Here's how the part is built. I have some questions about the finished solid (model axes, mm). A direction names the side the tool comes from. Round coordinates to 2 decimals unless told otherwise and drop trailing zeros. Write each loop counter-clockwise with the first axis right and the second up, starting at its lowest first coordinate (ties: lowest second). Pieces come first, ordered by that corner, then holes. Notation, with made-up numbers: (65.25, 72) -> (82.25, 72) arc R23 cw to (82.25, 88) -> close; hole circle Ø4 at (-21.5, 38). An arc over 180 degrees is marked (long way). Put each result on its own line as item: value. Start each with the question number.
1) I want a section at A-A, the plane x = 28.5. List the corners of the cut face in (y, z) for me.
2) I want a section at C-C, the plane y = 7. List the corners of the cut face in (x, z) for me.
3) I want a section at D-D, the plane x = 16.5. List the corners of the cut face in (y, z) for me, then the cut area to 3 significant figures.
4) Which directions (+Z, -Z, +X, -X, +Y, -Y) give clear straight access to the entire face, cutting with the end or side of a thin tool? Please do faces 5 (the flat face through (24.088, -24, 2)), 6 (the flat face through (32.004, -19, 2)), 7 (the flat face through (30, 16.002, 2)), 8 (the flat face through (12.817, -23, 2)), 9 (the flat face through (19.202, 21, 2)).
5) Will these pins go through, and if not, where does the flat tip stop? P1, Ø1.4, axis at x = 26, z = 3, coming from the -Y side; P2, Ø1.6, axis at x = 6.5, z = 3, coming from the +Y side; P3, Ø1.4, axis at y = -12, z = 1.5, coming from the +X side.
6) We'd pull the mould along Y, two halves only. Please class faces 1 (the flat face through (5.98, -8, 2)), 2 (the flat face through (27.445, 11, 2)), 3 (the flat face through (30, 5.334, 2)), 4 (the flat face through (7, 3.272, 2)): released by +Y, released by -Y, zero draft, split by the parting line, or undercut.
7) If I drill on line 1 along Y through (x, z) = (29.25, 4.25); line 2 along X through (y, z) = (21, 1.45); line 3 along X through (y, z) = (-12, 0.3), over which ranges is the centre line in solid material (lowest first)? Write a range as [from, to].
8) I want a section at B-B, the plane z = 1.05. List the corners of the cut face in (x, y) for me.
from build123d import *

# Parameters (mm, degrees)
BOSS_EXTRUDE1_DEPTH = 4.5593


with BuildPart() as part:
    # Sketch1 → Boss-Extrude1 (new body)
    with BuildSketch(Plane.XY):
        Polygon((24.0884075, -21.336), (32.004, -21.336), (32.004, -16.002), (27.4447, -16.002), (27.4447, -5.334), (32.004, -5.334), (32.004, 5.334), (27.4447, 5.334), (27.4447, 16.002), (32.004, 16.002), (32.004, 26.67), (19.2024, 26.67), (19.2024, 21.336), (19.2024, 16.002), (7.47522, 16.002), (7.47522, 12.9921), (7.47522, 3.27152), (5.980176, 3.27152), (5.980176, -19.0119), (8.2572225, -19.0119), (12.8165225, -19.0119), (12.8165225, -26.67), (24.0884075, -26.67), align=None)
    extrude(amount=BOSS_EXTRUDE1_DEPTH)


solid = part.part
Findings:
1. outline: (-21.34, 0) -> (-16, 0) -> (-16, 4.56) -> (-21.34, 4.56) -> close; (-5.33, 0) -> (5.33, 0) -> (5.33, 4.56) -> (-5.33, 4.56) -> close; (16, 0) -> (26.67, 0) -> (26.67, 4.56) -> (16, 4.56) -> close
2. outline: (7.48, 0) -> (27.44, 0) -> (27.44, 4.56) -> (7.48, 4.56) -> close
3. outline: (-26.67, 0) -> (16, 0) -> (16, 4.56) -> (-26.67, 4.56) -> close
3. area: 195 mm2
4. face 5: +Z, -Z, +X, -Y
4. face 6: +Z, -Z, +X, +Y, -Y
4. face 7: +Z, -Z, +X
4. face 8: +Z, -Z, -X, -Y
4. face 9: +Z, -Z, -X, +Y
5. P1: stops at y = -21.34
5. P2: stops at y = 3.27
5. P3: stops at x = 27.44
6. face 1: zero draft
6. face 2: undercut
6. face 3: undercut
6. face 4: released by +Y
7. line 1: y = [-21.34, -16], [-5.33, 5.33], [16, 26.67]
7. line 2: x = [19.2, 32]
7. line 3: x = [5.98, 27.44]
8. outline: (5.98, -19.01) -> (12.82, -19.01) -> (12.82, -26.67) -> (24.09, -26.67) -> (24.09, -21.34) -> (32, -21.34) -> (32, -16) -> (27.44, -16) -> (27.44, -5.33) -> (32, -5.33) -> (32, 5.33) -> (27.44, 5.33) -> (27.44, 16) -> (32, 16) -> (32, 26.67) -> (19.2, 26.67) -> (19.2, 16) -> (7.48, 16) -> (7.48, 3.27) -> (5.98, 3.27) -> close
